Answer from the drawing. Dimensions are ordinates in mm from the lowest x, y and z of the part. A direction names the side the tool comes from. Round coordinates to 2 decimals unless told otherwise and drop trailing zeros. Write each loop counter-clockwise with the first axis right and the second up, starting at its lowest first coordinate (ties: lowest second). Pieces come first, ordered by that corner, then holes.
1. A tool of negligible diameter and unlimited length cuts with its end or side. For the marked faces 1 and 2, from which of +Z, -Z, +X, -X, +Y, -Y can it reach the whole face along a straight path? Write none if from no direction.
2. Find section B-B (z = 9). Write down the section's boundary in (x, y), and give its area (3 significant figures).
3. Flat-ended cylindrical pins translate along their axes: pin 1 Ø3.5 at (x, z) = (3, 9) entering from +Y; pin 2 Ø1 at (x, y) = (3.5, 3) entering from -Z; pin 3 Ø1.5 at (y, z) = (4, 7.5) entering from +X; pin 4 Ø2 at (y, z) = (1.5, 12.5) entering from +X. Find the tip coordinate at first contact, or state that the pin passes through.
4. Find section A-A (x = 9). Write down the section's boundary in (y, z) (3 decimals), and give its area (3 significant figures).
5. Find section D-D (x = 15.75). Write down the section's boundary in (y, z), and give its area (3 significant figures).
6. Find section C-C (y = 1.7). Write down the section's boundary in (x, z) (3 decimals).
7. Determine the mould class of the marked faces 3, 4 and 5 for opening direction X: pulls with the +X half, pulls with the -X half, needs draft (parallel to the pull), parting line crosses it, or undercut.
8. Straight lines are drawn through the part: probe 1 along Z at (x, y) = (6, 0.3) (3 decimals); probe 2 along X at (y, z) = (2.15, 8); probe 3 along Z at (x, y) = (1.75, 5.1). For each, find the intervals that lie inside material, in ascending order.
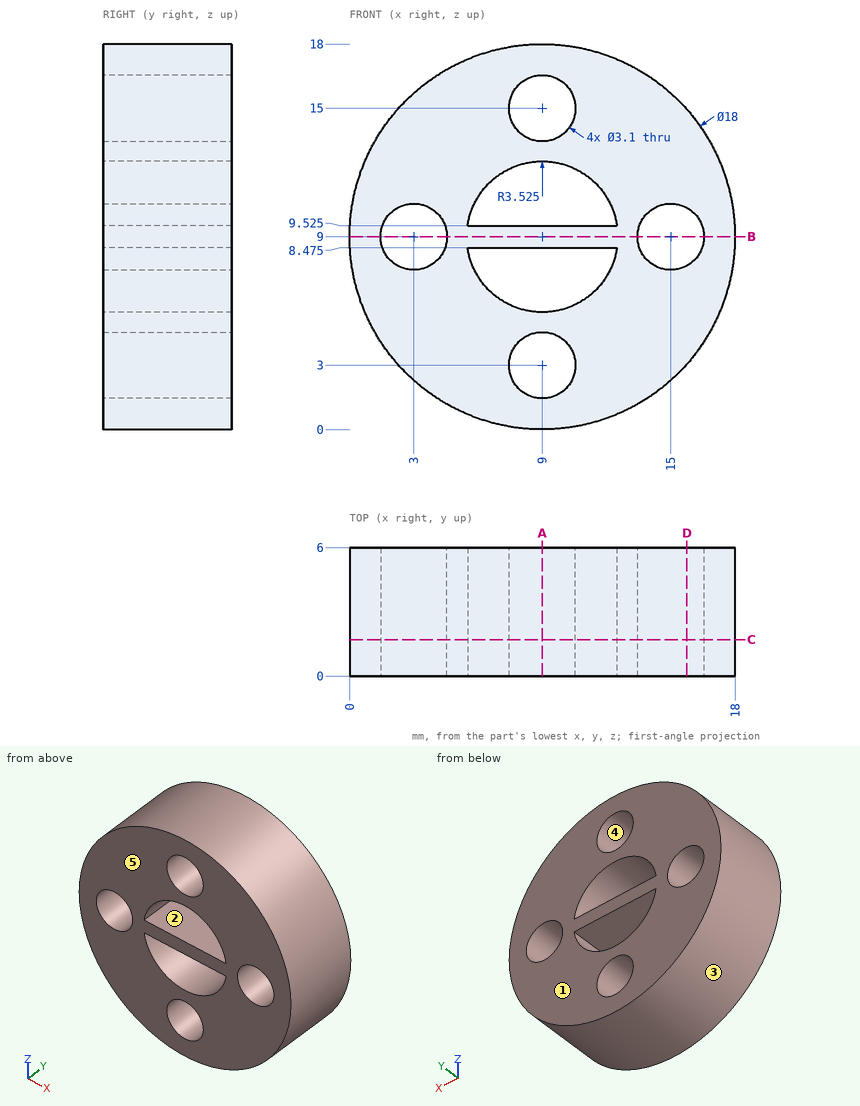
Worked answers:
1. face 1: +Z, -Z, +X, -X, +Y
1. face 2: +Y, -Y
2. outline: (0, 0) - (1.45, 0) - (1.45, 6) - (0, 6) - close; (4.55, 0) - (13.45, 0) - (13.45, 6) - (4.55, 6) - close; (16.55, 0) - (18, 0) - (18, 6) - (16.55, 6) - close
2. area: 70.8 mm2
3. pin 1: stops at y = 6
3. pin 2: stops at z = 1.52
3. pin 3: stops at x = 17.97
3. pin 4: stops at x = 17.65
4. outline: (0, 0) - (6, 0) - (6, 1.45) - (0, 1.45) - close; (0, 4.55) - (6, 4.55) - (6, 5.475) - (0, 5.475) - close; (0, 8.475) - (6, 8.475) - (6, 9.525) - (0, 9.525) - close; (0, 12.525) - (6, 12.525) - (6, 13.45) - (0, 13.45) - close; (0, 16.55) - (6, 16.55) - (6, 18) - (0, 18) - close
4. area: 34.8 mm2
5. outline: (0, 3.05) - (6, 3.05) - (6, 7.64) - (0, 7.64) - close; (0, 10.36) - (6, 10.36) - (6, 14.95) - (0, 14.95) - close
5. area: 55.2 mm2
6. outline: circle Ø18 at (9, 9); hole circle Ø3.1 at (3, 9); hole (5.514, 8.475) arc R3.525 ccw to (12.486, 8.475) - close; hole (5.514, 9.525) - (12.486, 9.525) arc R3.525 ccw to start; hole circle Ø3.1 at (9, 3); hole circle Ø3.1 at (9, 15); hole circle Ø3.1 at (15, 9)
7. face 3: parting line crosses it
7. face 4: undercut
7. face 5: needs draft
8. probe 1: z = 0.515 to 7.149, 8.475 to 9.525, 10.851 to 17.485
8. probe 2: x = 0.06 to 1.82, 4.18 to 5.62, 12.38 to 13.82, 16.18 to 17.94
8. probe 3: z = 3.67 to 8.08, 9.92 to 14.33
